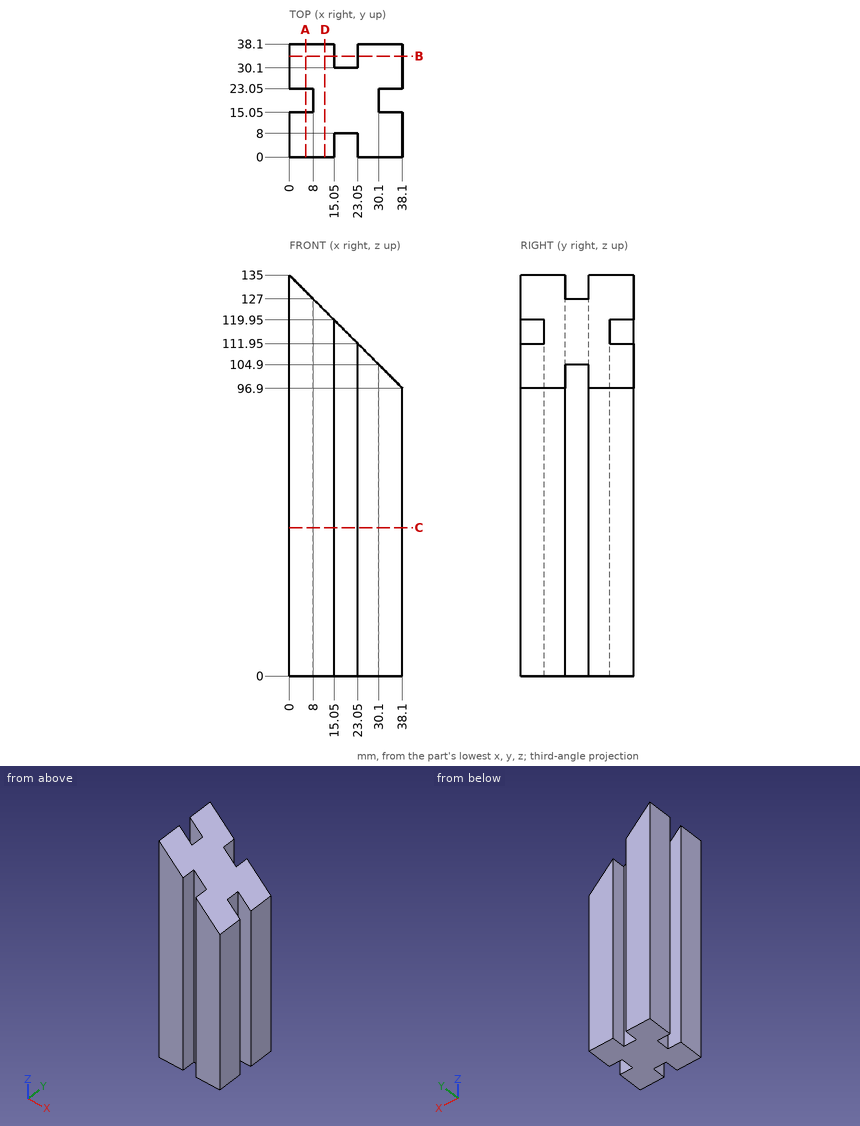
Design review of the part shown in the three views and the two pictorial views. Dimensions are in mm from the part's minimum x, y and z. Coordinates: 2 decimals unless noted, no trailing zeros. Order: outer loops, then holes, each group sorted by start corner. A loop starts at its lowest first (then second) coordinate and runs counter-clockwise, first axis right, second up.
Item 1: Take a section at B-B, the plane y = 34. Write out the cut boundary in (x, z), then the cut area to 3 significant figures.
Item 2: Take a section at C-C, the plane z = 50. Write out the cut boundary in (x, y), then the cut area to 3 significant figures.
Item 3: Take a section at D-D, the plane x = 12. Write out the cut boundary in (y, z).
Item 4: For pin 1 Ø4 at (y, z) = (18.5, 40) entering from +X; pin 2 Ø1.5 at (x, y) = (21.5, 13.5) entering from +Z; pin 3 Ø3 at (y, z) = (17.5, 112.5) entering from -X, all flat-tipped, find the tip position at first contact; note any pin that passes through.
Item 5: For line 1 (X direction, y = 4.5, z = 86); line 2 (Y direction, x = 20, z = 86.5), list the stretches that pass through material, from the lowest coordinate up.
Item 6: Take a section at A-A, the plane x = 5.5. Write out the cut boundary in (y, z), then the cut area to 3 significant figures.
The answers:
1. outline: (0, 0) - (15.05, 0) - (15.05, 119.95) - (0, 135) - close; (23.05, 0) - (38.1, 0) - (38.1, 96.9) - (23.05, 111.95) - close
1. area: 3,490 mm2
2. outline: (0, 0) - (15.05, 0) - (15.05, 8) - (23.05, 8) - (23.05, 0) - (38.1, 0) - (38.1, 15.05) - (30.1, 15.05) - (30.1, 23.05) - (38.1, 23.05) - (38.1, 38.1) - (23.05, 38.1) - (23.05, 30.1) - (15.05, 30.1) - (15.05, 38.1) - (0, 38.1) - (0, 23.05) - (8, 23.05) - (8, 15.05) - (0, 15.05) - close
2. area: 1,200 mm2
3. outline: (0, 0) - (38.1, 0) - (38.1, 123) - (0, 123) - close
4. pin 1: stops at x = 30.1
4. pin 2: stops at z = 114.25
4. pin 3: stops at x = 8
5. line 1: x = 0 to 15.05, 23.05 to 38.1
5. line 2: y = 8 to 30.1
6. outline: (0, 0) - (15.05, 0) - (15.05, 129.5) - (0, 129.5) - close; (23.05, 0) - (38.1, 0) - (38.1, 129.5) - (23.05, 129.5) - close
6. area: 3,900 mm2
